from build123d import *

# Parameters (mm, degrees)
BOSS_EXTRUDE1_DEPTH = 3.175
SKETCH3_R           = 2.54
CUT_EXTRUDE1_DEPTH  = 100.267219786


with BuildPart() as part:
    # Sketch2 → Boss-Extrude1 (new body)
    with BuildSketch(Plane(origin=(0, 0, 0), x_dir=(0, 0, -1), z_dir=(1, 0, 0))):
        with BuildLine():
            Line((60.967707714, -54.648816697), (5.189086512, 4.863530115))
            ThreePointArc((5.189086512, 4.863530115), (7.105260379, -0.309546352), (4.746461891, -5.296380228))
            Line((4.746461891, -5.296380228), (-0.432958039, -9.938025702))
            Line((-0.432958039, -9.938025702), (50.589534691, -64.375876927))
            ThreePointArc((50.589534691, -64.375876927), (60.642151317, -64.701433324), (60.967707714, -54.648816697))
        make_face()
        with BuildLine():
            ThreePointArc((-5.189086512, -4.863530115), (-7.105260379, 0.309546352), (-4.746461891, 5.296380228))
            Line((-4.746461891, 5.296380228), (-71.153824721, -54.215966584))
            ThreePointArc((-71.153824721, -54.215966584), (-71.703743057, -64.258808703), (-61.660900939, -64.80872704))
            Line((-61.660900939, -64.80872704), (-0.432958039, -9.938025702))
            Line((-0.432958039, -9.938025702), (-5.189086512, -4.863530115))
        make_face()
        with BuildLine():
            ThreePointArc((4.746461891, -5.296380228), (7.105260379, -0.309546352), (5.189086512, 4.863530115))
            ThreePointArc((5.189086512, 4.863530115), (0.309546352, 7.105260379), (-4.746461891, 5.296380228))
            ThreePointArc((-4.746461891, 5.296380228), (-7.105260379, 0.309546352), (-5.189086512, -4.863530115))
            Line((-5.189086512, -4.863530115), (-0.432958039, -9.938025702))
            Line((-0.432958039, -9.938025702), (4.746461891, -5.296380228))
        make_face()
    extrude(amount=BOSS_EXTRUDE1_DEPTH)

    # Sketch3 → Cut-Extrude1 (cut, through all)
    with BuildSketch(Plane(origin=(3.175, 0, 0), x_dir=(0, 0, -1), z_dir=(1, 0, 0))):
        Circle(SKETCH3_R)
        with Locations((-66.40736283, -59.512346812)):
            Circle(SKETCH3_R)
        with Locations((55.778621202, -59.512346812)):
            Circle(SKETCH3_R)
    extrude(amount=-CUT_EXTRUDE1_DEPTH, mode=Mode.SUBTRACT)


solid = part.part
Read the model definition and answer for the solid it produces. Units are mm, in the model's axes. A direction names the side the tool comes from. Round coordinates to 2 decimals unless told otherwise and drop trailing zeros. Loops run counter-clockwise (first coordinate to the right, second up) from the corner with the lowest first, then second, coordinate; pieces in that order, holes last. Notation, with made-up numbers: (42, 4) - (51, 4) arc R31 ccw to (51, 29) - close; hole circle Ø5 at (-15, 67.25). An arc over 180 degrees is marked (long way). One line per question, with ' | ' between items. Start each with the question number.
Q1. For faces 1 (the flat face through (3.175, -21, 16)), 2 (the flat face through (1.565, -36.776, -24.721)), determine the directions among +Z, -Z, +X, -X, +Y, -Y from which every point of the face is accessible in a straight line to the end or side of a thin tool.
Q2. Section C-C on y = -34 is taken. Give the vertices of the cut face in (x, z) (3 decimals).
Q3. Find the intervals of material crossed by L1, parallel to Z at x = 1.1, y = -58; L2, parallel to Z at x = 1.8, y = -13.5; L3, parallel to Z at x = 2.6, y = -50.5, in increasing order.
Q4. Section D-D on z = -6.5 is taken. Give the vertices of the cut face in (x, y) (3 decimals).
Q5. Section A-A on y = 0 is taken. Give the vertices of the cut face in (x, z) (3 decimals), plus the area to 3 significant figures.
Q6. Section B-B on x = 1.45 is taken. Give the vertices of the cut face in (y, z), plus the area to 3 significant figures.
Q7. For a pull along Z with two mould halves and no side action, classify faces 3 (the flat face through (0, -21, 16)), 4 (the cylindrical face through (1.6, 7.1, -0.4)), 5 (the flat face through (1.57, -37.76, 31.48)) as +Z half, -Z half, draft (parallel to the pull), parting line (faces both ways), or undercut.
Q8. Flat-ended cylindrical pins translate along their axes: pin 1 (1 mm diameter, centred on x = 0.5, y = -35, fed in from +Z); pin 2 (1.5 mm diameter, centred on x = 1.5, z = -36.5, fed in from -Y); pin 3 (1 mm diameter, centred on x = 1, y = -39, fed in from -Z). Find the tip coordinate at first contact, or state that the pin passes through.
Established:
1) face 1: +Z, -Z, +X, +Y, -Y | face 2: +X, -X, -Y
2) outline: (0, -41.614) - (3.175, -41.614) - (3.175, -22.119) - (0, -22.119) - close; (0, 27.283) - (3.175, 27.283) - (3.175, 48.596) - (0, 48.596) - close
3) L1: -62.73 to -57.82, -53.74 to -44.61, 54.06 to 64.37, 68.45 to 73.36 | L2: -22.4 to -2.91, 4.41 to 25.72 | L3: -57.08 to -37.58, 45.69 to 67.01
4) outline: (0, -17.335) - (3.175, -17.335) - (3.175, 3.465) - (0, 3.465) - close
5) outline: (0, -9.747) - (3.175, -9.747) - (3.175, -2.54) - (0, -2.54) - close; (0, 2.54) - (3.175, 2.54) - (3.175, 10.656) - (0, 10.656) - close | area: 48.7 mm²
6) outline: (-64.81, 61.66) - (-9.94, 0.43) - (-64.38, -50.59) arc R7.11 ccw to (-54.65, -60.97) - (4.86, -5.19) arc R7.11 ccw to (5.3, 4.75) - (-54.22, 71.15) arc R7.11 ccw to start; hole circle Ø5.08 at (-59.51, -55.78); hole circle Ø5.08 at (-59.51, 66.41); hole circle Ø5.08 at (0, 0) | area: 2,520 mm²
7) face 3: draft | face 4: parting line | face 5: undercut
8) pin 1: z = 50.27 | pin 2: y = -50.14 | pin 3: z = -46.77
